Verification items for this drawing (mm, ordinates from the low corner). Round coordinates to 2 decimals unless told otherwise and drop trailing zeros. Loops run counter-clockwise (first coordinate to the right, second up) from the corner with the lowest first, then second, coordinate; pieces in that order, holes last. Notation, with made-up numbers: (9, -3.5) -> (27, -3.5) arc R30 ccw to (27, 31.5) -> close; hole circle Ø7 at (-31.75, -24.75). An arc over 180 degrees is marked (long way). One line per item, written item: value. Start each with the question number.
1. Go/stop test with flat-tipped pins: pin 1 (5 mm diameter, centred on x = 9.5, y = 27.5, fed in from -Z); pin 2 (1.5 mm diameter, centred on x = 4, z = 2.5, fed in from +Y) (1 decimal); pin 3 (0.8 mm diameter, centred on x = 0.5, z = 1.5, fed in from -Y); pin 4 (1.5 mm diameter, centred on y = 8.5, z = 0.5, fed in from +X). Record where each tip stops, or that it passes through.
2. Cross-section at B-B on x = 3. Record the cut outline in (y, z) (1 decimal).
3. Cross-section at C-C on z = 1.25. Count the separate pieces of the cut face and the enclosed holes in it, then the cut area to 3 significant figures.
4. Material ranges on L1, parallel to X at y = 13, z = 1.75; L2, parallel to X at y = 50, z = 2.45; L3, parallel to X at y = 5.5, z = 1.7 (1 decimal), recorded low to high.
5. Cross-section at A-A on y = 5. Record the cut outline in (x, z).
6. Cross-section at D-D on x = 25. Record the cut outline in (y, z) (1 decimal).
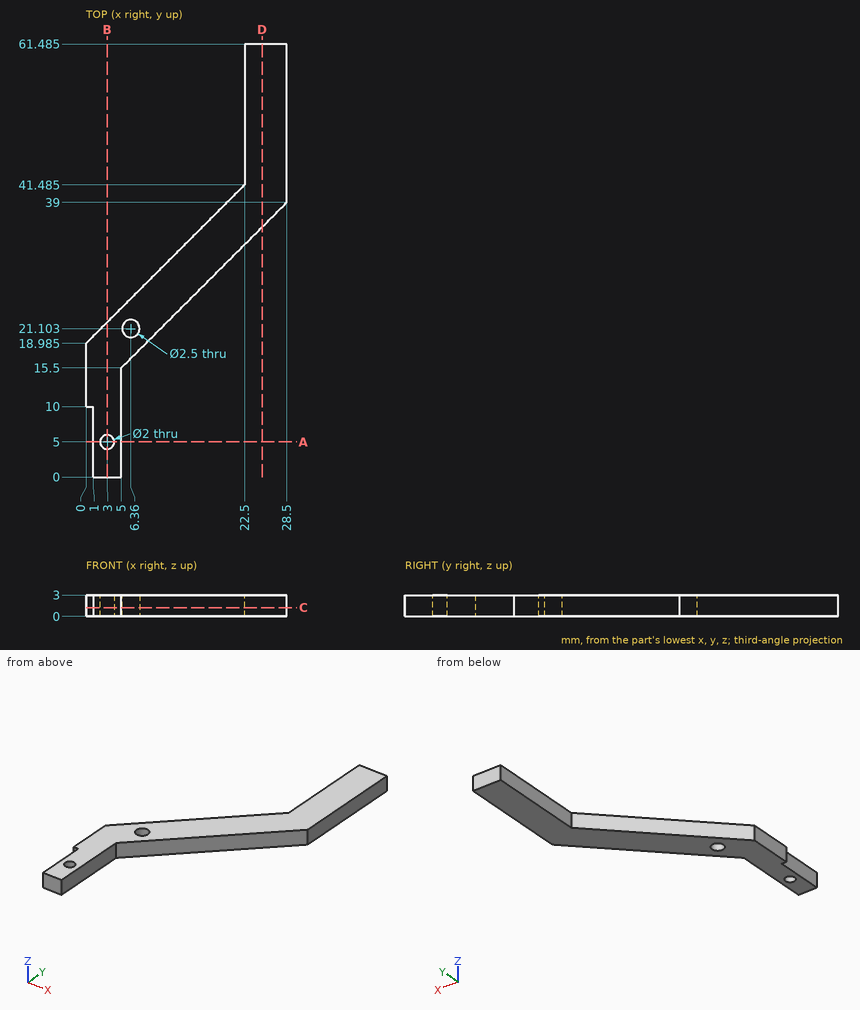
Taken from the geometry:
1. pin 1: stops at z = 0
1. pin 2: stops at y = 23.7
1. pin 3: stops at y = 10
1. pin 4: stops at x = 5
2. outline: (0, 0) -> (4, 0) -> (4, 3) -> (0, 3) -> close; (6, 0) -> (22, 0) -> (22, 3) -> (6, 3) -> close
3. separate pieces: 1
3. enclosed holes: 2
3. area: 391 mm2
4. L1: x = 0 to 5
4. L2: x = 22.5 to 28.5
4. L3: x = 1 to 2.1, 3.9 to 5
5. outline: (1, 0) -> (2, 0) -> (2, 3) -> (1, 3) -> close; (4, 0) -> (5, 0) -> (5, 3) -> (4, 3) -> close
6. outline: (35.5, 0) -> (61.5, 0) -> (61.5, 3) -> (35.5, 3) -> close
